```python
from build123d import *

# Parameters (mm, degrees)
SKETCH2_R             = 30.880396168
HUB_DEPTH             = 14
SKETCH4_R             = 1.6
AXLE_AND_SCREWS_DEPTH = 15
RIBS_REACH            = 16


with BuildPart() as part:
    # Sketch2 → Hub (new body)
    with BuildSketch(Plane.XY):
        Circle(SKETCH2_R)
    extrude(amount=HUB_DEPTH)

    # Sketch4 → Axle and screws (cut, through all)
    with BuildSketch(Plane.XY):
        with Locations((12.940198084, -22.413080541)):
            Circle(SKETCH4_R)
        with Locations((-12.940198084, -22.413080541)):
            Circle(SKETCH4_R)
        with Locations((-25.880396168, 0)):
            Circle(SKETCH4_R)
        with Locations((-12.940198084, 22.413080541)):
            Circle(SKETCH4_R)
        with Locations((12.940198084, 22.413080541)):
            Circle(SKETCH4_R)
        with Locations((25.880396168, 0)):
            Circle(SKETCH4_R)
        Polygon((-1.890822132, -3.275), (1.890822132, -3.275), (3.781644263, 0), (1.890822132, 3.275), (-1.890822132, 3.275), (-3.781644263, 0), align=None)
    extrude(amount=AXLE_AND_SCREWS_DEPTH, mode=Mode.SUBTRACT)

    # Sketch5 → Ribs (cut, up to next)
    with BuildSketch(Plane.XY, mode=Mode.PRIVATE) as ribs_sk1:
        with BuildLine():
            Line((-5.434309409, -3.1375), (-20.643329137, -3.1375))
            ThreePointArc((-20.643329137, -3.1375), (-18.082953522, -10.440198084), (-13.038819273, -16.308897452))
            Line((-13.038819273, -16.308897452), (-5.434309409, -3.1375))
        make_face()
    ribs_tool1 = extrude(ribs_sk1.sketch, amount=RIBS_REACH, mode=Mode.PRIVATE) & part.part
    add(ribs_tool1.solids().sort_by_distance((-13.587324, -7.844645, 0))[0], mode=Mode.SUBTRACT)
    # Sketch5 → Ribs (cut, up to next)
    with BuildSketch(Plane.XY, mode=Mode.PRIVATE) as ribs_sk2:
        with BuildLine():
            Line((0, -6.275), (-7.604509864, -19.446397452))
            ThreePointArc((-7.604509864, -19.446397452), (0, -20.880396168), (7.604509864, -19.446397452))
            Line((7.604509864, -19.446397452), (0, -6.275))
        make_face()
    ribs_tool2 = extrude(ribs_sk2.sketch, amount=RIBS_REACH, mode=Mode.PRIVATE) & part.part
    add(ribs_tool2.solids().sort_by_distance((0, -15.68929, 0))[0], mode=Mode.SUBTRACT)
    # Sketch5 → Ribs (cut, up to next)
    with BuildSketch(Plane.XY, mode=Mode.PRIVATE) as ribs_sk3:
        with BuildLine():
            Line((5.434309409, -3.1375), (13.038819273, -16.308897452))
            ThreePointArc((13.038819273, -16.308897452), (18.082953522, -10.440198084), (20.643329137, -3.1375))
            Line((20.643329137, -3.1375), (5.434309409, -3.1375))
        make_face()
    ribs_tool3 = extrude(ribs_sk3.sketch, amount=RIBS_REACH, mode=Mode.PRIVATE) & part.part
    add(ribs_tool3.solids().sort_by_distance((13.587324, -7.844645, 0))[0], mode=Mode.SUBTRACT)
    # Sketch5 → Ribs (cut, up to next)
    with BuildSketch(Plane.XY, mode=Mode.PRIVATE) as ribs_sk4:
        with BuildLine():
            Line((5.434309409, 3.1375), (20.643329137, 3.1375))
            ThreePointArc((20.643329137, 3.1375), (18.082953522, 10.440198084), (13.038819273, 16.308897452))
            Line((13.038819273, 16.308897452), (5.434309409, 3.1375))
        make_face()
    ribs_tool4 = extrude(ribs_sk4.sketch, amount=RIBS_REACH, mode=Mode.PRIVATE) & part.part
    add(ribs_tool4.solids().sort_by_distance((13.587324, 7.844645, 0))[0], mode=Mode.SUBTRACT)
    # Sketch5 → Ribs (cut, up to next)
    with BuildSketch(Plane.XY, mode=Mode.PRIVATE) as ribs_sk5:
        with BuildLine():
            Line((-20.643329137, 3.1375), (-5.434309409, 3.1375))
            Line((-5.434309409, 3.1375), (-13.038819273, 16.308897452))
            ThreePointArc((-13.038819273, 16.308897452), (-18.082953522, 10.440198084), (-20.643329137, 3.1375))
        make_face()
    ribs_tool5 = extrude(ribs_sk5.sketch, amount=RIBS_REACH, mode=Mode.PRIVATE) & part.part
    add(ribs_tool5.solids().sort_by_distance((-13.587324, 7.844645, 0))[0], mode=Mode.SUBTRACT)
    # Sketch5 → Ribs (cut, up to next)
    with BuildSketch(Plane.XY, mode=Mode.PRIVATE) as ribs_sk6:
        with BuildLine():
            Line((0, 6.275), (7.604509864, 19.446397452))
            ThreePointArc((7.604509864, 19.446397452), (0, 20.880396168), (-7.604509864, 19.446397452))
            Line((-7.604509864, 19.446397452), (0, 6.275))
        make_face()
    ribs_tool6 = extrude(ribs_sk6.sketch, amount=RIBS_REACH, mode=Mode.PRIVATE) & part.part
    add(ribs_tool6.solids().sort_by_distance((0, 15.68929, 0))[0], mode=Mode.SUBTRACT)


solid = part.part
```
Check sheet for the modelled part. Datum: model origin and axes. Units: mm. Coordinates: 2 decimals unless noted, no trailing zeros. Loops run counter-clockwise (first coordinate to the right, second up) from the corner with the lowest first, then second, coordinate; pieces in that order, holes last.
1) Material ranges on probe 1 along X at (y, z) = (4, 6.75); probe 2 along X at (y, z) = (-21.5, 1.25); probe 3 along X at (y, z) = (6.5, 8.25), recorded low to high.
2) Release check for a two-part mould opening along Y. For faces 1 (the face through (0, -6, 14)), 2 (the face through (29.454, 9.276, 6.902)), 3 (the face through (0.11, 20.88, 6.9)), 4 (the face through (13, 3.138, 7)) record: released by +Y, released by -Y, zero draft, split by the parting line, or undercut.
3) Sectioned sample at A-A (y = -9). Record the boundary of the cut face in (x, z).
4) Gauge pin test, flat ends, axial feed: pin 1 (7 mm diameter, centred on x = 14, z = 7.5, fed in from -Y); pin 2 (1.5 mm diameter, centred on x = -16, y = 9, fed in from -Z); pin 3 (1.9 mm diameter, centred on x = 0.5, z = 10.5, fed in from +Y); pin 4 (4 mm diameter, centred on x = -10, z = 4.5, fed in from +Y). Record the tip position at first contact, or that the pin passes through.
5) Sectioned sample at B-B (x = 17.5). Record the boundary of the cut face in (y, z).
6) Sectioned sample at C-C (y = 17.5). Record the boundary of the cut face in (x, z).
7) Sectioned sample at D-D (z = 7.75). Count the separate pieces of the cut face and the enclosed holes in it, and give its area (3 significant figures).
Check sheet entries:
1. probe 1: x = -30.62 to -20.49, -5.93 to 5.93, 20.49 to 30.62
1. probe 2: x = -22.17 to -14.25, -11.63 to 11.63, 14.25 to 22.17
1. probe 3: x = -30.19 to -19.84, -7.38 to -0.13, 0.13 to 7.38, 19.84 to 30.19
2. face 1: zero draft
2. face 2: split by the parting line
2. face 3: undercut
2. face 4: undercut
3. outline: (-29.54, 0) - (-18.84, 0) - (-18.84, 14) - (-29.54, 14) - close; (-8.82, 0) - (-1.57, 0) - (-1.57, 14) - (-8.82, 14) - close; (1.57, 0) - (8.82, 0) - (8.82, 14) - (1.57, 14) - close; (18.84, 0) - (29.54, 0) - (29.54, 14) - (18.84, 14) - close
4. pin 1: stops at y = -29.04
4. pin 2: passes through
4. pin 3: stops at y = 30.88
4. pin 4: stops at y = 29.83
5. outline: (-25.44, 0) - (-11.39, 0) - (-11.39, 14) - (-25.44, 14) - close; (-3.14, 0) - (3.14, 0) - (3.14, 14) - (-3.14, 14) - close; (11.39, 0) - (25.44, 0) - (25.44, 14) - (11.39, 14) - close
6. outline: (-25.44, 0) - (-6.48, 0) - (-6.48, 14) - (-25.44, 14) - close; (6.48, 0) - (25.44, 0) - (25.44, 14) - (6.48, 14) - close
7. separate pieces: 1
7. enclosed holes: 13
7. area: 2,220 mm2
